For this review, take the finished solid that the model builds, in its own axes (mm). A direction names the side the tool comes from. Round coordinates to 2 decimals unless told otherwise and drop trailing zeros. Write each loop counter-clockwise with the first axis right and the second up, starting at its lowest first coordinate (ties: lowest second). Pieces come first, ordered by that corner, then holes. Notation, with made-up numbers: M -12.75,60.5 L 22.25,60.5 A13 ccw 22.25,84.5 Z; hole C 47,33.5 d5. An arc over 180 degrees is marked long. Answer in a Markdown table with one row per item.
```python
from build123d import *

# Parameters (mm, degrees)
F1_DEPTH = 20
F2_DEPTH = 10


with BuildPart() as f1:
    # F0 (on Front) → F1 (new body)
    with BuildSketch(Plane.XZ):
        with BuildLine():
            Line((0.7485, 20.5), (1.072906, 22.474405))
            ThreePointArc((1.072906, 22.474405), (0, 22.5), (-1.072906, 22.474405))
            Line((-1.072906, 22.474405), (-0.7485, 20.5))
            Line((-0.7485, 20.5), (0.7485, 20.5))
        make_face()
        with BuildLine():
            ThreePointArc((-1.072906, 22.474405), (0, 22.5), (1.072906, 22.474405))
            Line((1.072906, 22.474405), (1.12626, 22.799129))
            Line((1.12626, 22.799129), (-1.12626, 22.799129))
            Line((-1.12626, 22.799129), (-1.072906, 22.474405))
        make_face()
    extrude(amount=F1_DEPTH)

    # F0 (on Front) → F2 (join)
    with BuildSketch(Plane.XZ):
        with BuildLine():
            ThreePointArc((-1.072906, 22.474405), (-15.52594, -16.284815), (22.5, 0))
            ThreePointArc((22.5, 0), (16.284815, 15.52594), (1.072906, 22.474405))
            Line((1.072906, 22.474405), (0.7485, 20.5))
            Line((0.7485, 20.5), (-0.7485, 20.5))
            Line((-0.7485, 20.5), (-1.072906, 22.474405))
        make_face()
    extrude(amount=F2_DEPTH)


solid = f1.part
```
Q1. For probe 1 along Y at (x, z) = (18, -6); probe 2 along Z at (x, y) = (-16, -4); probe 3 along X at (y, z) = (-6.5, -16.5), list the stretches that pass through material, from the lowest coordinate up.
Found:
| item | result |
|---|---|
| probe 1 | -10 to 0 |
| probe 2 | -15.82 to 15.82 |
| probe 3 | -15.3 to 15.3 |
Q2. Insertion check: P1, Ø1.2, axis at x = 0, y = -13.5, coming from the -Z side; P2, Ø6, axis at y = -3.5, z = -4, coming from the -X side; P3, Ø8, axis at y = -10, z = 8.5, coming from the +X side. Each pin has a flat end and moves straight along its axis. Give the tip position at first contact, or say it passes through.
Found:
| item | result |
|---|---|
| P1 | z = 20.5 |
| P2 | x = -22.48 |
| P3 | x = 22.05 |
Q3. Take a section at A-A (y = -13.75). State the section outline as (x, z) points, then the cut area to 3 significant figures.
Found:
| item | result |
|---|---|
| outline | M -1.13,22.8 L -0.75,20.5 L 0.75,20.5 L 1.13,22.8 Z |
| area | 4.31 mm² |
Q4. Take a section at B-B (x = 19). State the section outline as (y, z) points, then the cut area to 3 significant figures.
Found:
| item | result |
|---|---|
| outline | M -10,-12.05 L 0,-12.05 L 0,12.05 L -10,12.05 Z |
| area | 241 mm² |
Q5. Machinability: for faces 1 (the face through (0, -15, 20.5)), 2 (the face through (0, 0, 0)), which of the approach directions +Z, -Z, +X, -X, +Y, -Y give a long, thin tool a straight path to every point of the face, cutting with its end or side? Answer none if there is none.
Found:
| item | result |
|---|---|
| face 1 | -Z, +X, -X, -Y |
| face 2 | +Z, -Z, +X, -X, +Y |
Q6. Take a section at D-D (y = -2). State the section outline as (x, z) points, then the cut area to 3 significant figures.
Found:
| item | result |
|---|---|
| outline | M -1.13,22.8 L -1.07,22.47 A22.5 ccw long 1.07,22.47 L 1.13,22.8 Z |
| area | 1,590 mm² |
Q7. Take a section at C-C (z = 11.5). State the section outline as (x, y) points.
Found:
| item | result |
|---|---|
| outline | M -19.34,-10 L 19.34,-10 L 19.34,0 L -19.34,0 Z |
